```python
from build123d import *

# Parameters (mm, degrees)
SKETCH1_W           = 20
SKETCH1_H           = 40
BOSS_EXTRUDE1_DEPTH = 3
SKETCH2_R           = 2.5
BOSS_EXTRUDE2_DEPTH = 7
CHAMFER1_SIZE       = 1
CHAMFER2_SIZE       = 0.5


with BuildPart() as part:
    # Sketch1 → Boss-Extrude1 (new body)
    with BuildSketch(Plane.XY):
        with Locations((10, 20)):
            Rectangle(SKETCH1_W, SKETCH1_H)
    extrude(amount=BOSS_EXTRUDE1_DEPTH)

    # Sketch2 → Boss-Extrude2 (add)
    with BuildSketch(Plane.XY.offset(3)):
        with Locations(Location((10, 30, 0), (0, 0, 180))):
            Circle(SKETCH2_R)
        with Locations(Location((10, 10, 0), (0, 0, 180))):
            Circle(SKETCH2_R)
    extrude(amount=BOSS_EXTRUDE2_DEPTH)

    # Chamfer1
    chamfer1_edges = [part.edges().sort_by_distance(p)[0] for p in [
        (12.5, 30, 10),
        (12.5, 10, 10),
    ]]
    chamfer(chamfer1_edges, length=CHAMFER1_SIZE)

    # Chamfer2
    chamfer2_edges = [part.edges().sort_by_distance(p)[0] for p in [
        (0, 40, 1.5),
        (20, 40, 1.5),
        (20, 0, 1.5),
        (0, 0, 1.5),
    ]]
    chamfer(chamfer2_edges, length=CHAMFER2_SIZE)


solid = part.part
```
Can you work these out from the model? Positions are in its coordinate system, mm. A direction names the side the tool comes from. Coordinates: 2 decimals unless noted, no trailing zeros. Order: outer loops, then holes, each group sorted by start corner. A loop starts at its lowest first (then second) coordinate and runs counter-clockwise, first axis right, second up.
1. If we section it at A-A (x = 10): Please give me the cut outline in (y, z).
2. If we section it at C-C (z = 8.5): Please give me the cut outline in (x, y).
3. I need wall thicknesses on line 1 (Z direction, x = 18, y = 5.5); line 2 (Y direction, x = 9.5, z = 4.75); line 3 (X direction, y = 10, z = 5.25). Which ranges of each line are inside material? Lowest first, please.
4. Thinking about a two-plate mould opening in Y: for faces 1 (the face through (10, 10, 10)), 2 (the face through (10, 0, 1)), 3 (the face through (10.54, 12.44, 5.96)), which applies, +Y half, -Y half, draft (parallel to the pull), parting line (faces both ways), or undercut?
5. For faces 4 (the face through (10.33, 27.52, 5.96)), 5 (the face through (10, 40, 1)), which set-ups out of +Z, -Z, +X, -X, +Y, -Y let a thin tool reach every point of the face, with its end or its side?
6. I'm going to push flat-ended pins straight in: pin 1 (3 mm diameter, centred on y = 10.5, z = 7, fed in from -X); pin 2 (1 mm diameter, centred on y = 8.5, z = 9, fed in from +X); pin 3 (10 mm diameter, centred on x = 9, y = 12.5, fed in from +Z). Where does each tip first touch, or does it pass through?
7. If we section it at D-D (x = 2.5): Please give me the cut outline in (y, z).
8. If we section it at B-B (y = 10): Please give me the cut outline in (x, z).
Entries:
1. outline: (0, 0) - (40, 0) - (40, 3) - (32.5, 3) - (32.5, 9) - (31.5, 10) - (28.5, 10) - (27.5, 9) - (27.5, 3) - (12.5, 3) - (12.5, 9) - (11.5, 10) - (8.5, 10) - (7.5, 9) - (7.5, 3) - (0, 3) - close
2. outline: circle Ø5 at (10, 10); circle Ø5 at (10, 30)
3. line 1: z = 0 to 3
3. line 2: y = 7.55 to 12.45, 27.55 to 32.45
3. line 3: x = 7.5 to 12.5
4. face 1: draft
4. face 2: -Y half
4. face 3: undercut
5. face 4: +Z
5. face 5: +Z, -Z, +X, -X, +Y
6. pin 1: stops at x = 7.5
6. pin 2: stops at x = 12.29
6. pin 3: stops at z = 10
7. outline: (0, 0) - (40, 0) - (40, 3) - (0, 3) - close
8. outline: (0, 0) - (20, 0) - (20, 3) - (12.5, 3) - (12.5, 9) - (11.5, 10) - (8.5, 10) - (7.5, 9) - (7.5, 3) - (0, 3) - close
